```python
from build123d import *

# Parameters (mm, degrees)
F0_R     = 75
F1_DEPTH = 40
F2_R     = 10
F3_R     = 10
F4_R     = 30
F5_DEPTH = 45
F6_R     = 5


with BuildPart() as f1:
    # F0 (on Front) → F1 (new body)
    with BuildSketch(Plane.XZ):
        Circle(F0_R)
    extrude(amount=F1_DEPTH)

    # F2
    f2_edges = [f1.edges().sort_by_distance(p)[0] for p in [
        (-75, -40, 0),
    ]]
    fillet(f2_edges, radius=F2_R)

    # F3
    f3_edges = [f1.edges().sort_by_distance(p)[0] for p in [
        (-75, 0, 0),
    ]]
    fillet(f3_edges, radius=F3_R)

    # F4 (on face) → F5 (cut)
    with BuildSketch(Plane(origin=(0, 0, 0), x_dir=(-1, 0, 0), z_dir=(0, 1, 0))):
        Circle(F4_R)
    extrude(amount=-F5_DEPTH, mode=Mode.SUBTRACT)

    # F6
    f6_edges = [f1.edges().sort_by_distance(p)[0] for p in [
        (30, -40, 0),
        (30, 0, 0),
    ]]
    fillet(f6_edges, radius=F6_R)


solid = f1.part
```
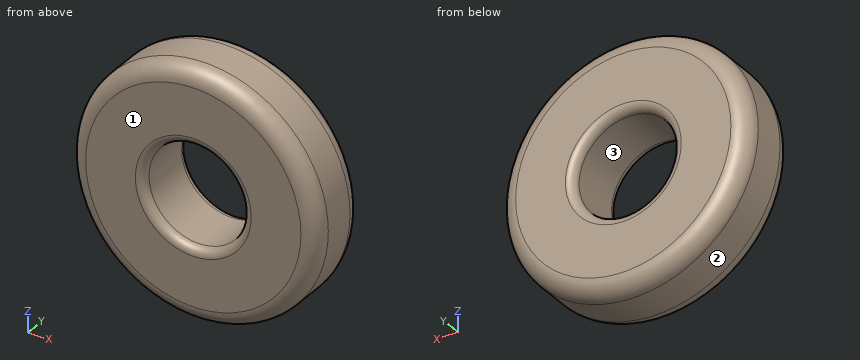
Check sheet for the modelled part. Datum: model origin and axes. Units: mm. Face numbers are marked on the shaded views. Give positions to 0.01 mm unless a question says otherwise; leave off trailing zeros. Write each loop counter-clockwise with the first axis right and the second up, starting at its lowest first coordinate (ties: lowest second). Pieces come first, ordered by that corner, then holes.
Item 1: Cross-section at D-D (y = -33). Enter the section's corners in (x, z), and give its area (3 significant figures).
Item 2: Cross-section at A-A (z = 0). Enter the section's corners in (x, y).
Item 3: Cross-section at C-C (y = -22.5). Enter the section's corners in (x, z).
Item 4: Scan lines: L1, parallel to Z at x = 0, y = -25.75; L2, parallel to Z at x = -5.5, y = -35; L3, parallel to X at y = -14.5, z = 3. Record each from-to range of solid material in increasing order.
Item 5: Cross-section at B-B (x = 0). Enter the section's corners in (y, z).
Item 6: Draft check along X on the marked faces 1, 2 and 3. Enter one of: released by +X, released by -X, zero draft, split by the parting line, or undercut.
Item 7: Gauge pin test, flat ends, axial feed: pin 1 (4 mm diameter, centred on x = 6.5, y = -24.5, fed in from -Z); pin 2 (4 mm diameter, centred on y = -7.5, z = 5, fed in from -X); pin 3 (3 mm diameter, centred on y = -22, z = -37.5, fed in from +X); pin 4 (8 mm diameter, centred on x = -44.5, z = 33.5, fed in from +Y). Record the tip position at first contact, or that the pin passes through.
Report:
1. outline: circle Ø149.08 at (0, 0); hole circle Ø60 at (0, 0)
1. area: 14,600 mm2
2. outline: (-75, -30) arc R10 ccw to (-65, -40) - (-35, -40) arc R5 ccw to (-30, -35) - (-30, -5) arc R5 ccw to (-35, 0) - (-65, 0) arc R10 ccw to (-75, -10) - close; (30, -35) arc R5 ccw to (35, -40) - (65, -40) arc R10 ccw to (75, -30) - (75, -10) arc R10 ccw to (65, 0) - (35, 0) arc R5 ccw to (30, -5) - close
3. outline: circle Ø150 at (0, 0); hole circle Ø60 at (0, 0)
4. L1: z = -75 to -30, 30 to 75
4. L2: z = -73.45 to -29.49, 29.49 to 73.45
4. L3: x = -74.94 to -29.85, 29.85 to 74.94
5. outline: (-40, -65) arc R10 ccw to (-30, -75) - (-10, -75) arc R10 ccw to (0, -65) - (0, -35) arc R5 ccw to (-5, -30) - (-35, -30) arc R5 ccw to (-40, -35) - close; (-40, 35) arc R5 ccw to (-35, 30) - (-5, 30) arc R5 ccw to (0, 35) - (0, 65) arc R10 ccw to (-10, 75) - (-30, 75) arc R10 ccw to (-40, 65) - close
6. face 1: zero draft
6. face 2: split by the parting line
6. face 3: undercut
7. pin 1: stops at z = -74.86
7. pin 2: stops at x = -74.86
7. pin 3: stops at x = 65.8
7. pin 4: stops at y = 0
